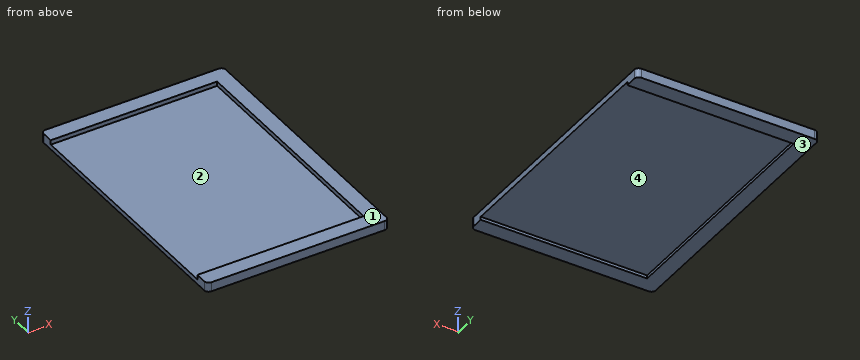
```python
from build123d import *

# Parameters (mm, degrees)
F1_DEPTH = 3.429
F3_DEPTH = 1.651
F5_DEPTH = 1.143


with BuildPart() as f1:
    # F0 (on Top) → F1 (new body)
    with BuildSketch(Plane.XY):
        with BuildLine():
            Line((-31.75, -49.022), (31.75, -49.022))
            ThreePointArc((31.75, -49.022), (32.872532, -48.557032), (33.3375, -47.4345))
            Line((33.3375, -47.4345), (33.3375, 47.4345))
            ThreePointArc((33.3375, 47.4345), (32.872532, 48.557032), (31.75, 49.022))
            Line((31.75, 49.022), (-31.75, 49.022))
            ThreePointArc((-31.75, 49.022), (-32.872532, 48.557032), (-33.3375, 47.4345))
            Line((-33.3375, 47.4345), (-33.3375, -47.4345))
            ThreePointArc((-33.3375, -47.4345), (-32.872532, -48.557032), (-31.75, -49.022))
        make_face()
    extrude(amount=F1_DEPTH)

    # F2 (on face) → F3 (cut)
    with BuildSketch(Plane.XY.offset(3.429)):
        Polygon((-27.6225, -43.307), (27.6225, -43.307), (27.6225, 43.307), (-27.6225, 43.307), (-33.3375, 43.307), (-33.3375, -43.307), align=None)
    extrude(amount=-F3_DEPTH, mode=Mode.SUBTRACT)

    # F4 (on face) → F5 (cut)
    with BuildSketch(Plane(origin=(0, 0, 0), x_dir=(1, 0, 0), z_dir=(0, 0, -1))):
        Polygon((-27.6225, -43.307), (27.6225, -43.307), (33.3375, -43.307), (33.3375, 43.307), (27.6225, 43.307), (-27.6225, 43.307), align=None)
    extrude(amount=-F5_DEPTH, mode=Mode.SUBTRACT)


solid = f1.part
```
Design review of the part built by this model. Coordinates are the model's own, in mm. Face numbers are marked on the shaded views. A direction names the side the tool comes from. Round coordinates to 2 decimals unless told otherwise and drop trailing zeros. Order: outer loops, then holes, each group sorted by start corner. A loop starts at its lowest first (then second) coordinate and runs counter-clockwise, first axis right, second up. Notation, with made-up numbers: (43.25, 3) - (53.25, 3) arc R17 cw to (53.25, 34) - close; hole circle Ø3 at (76.25, 33.5). An arc over 180 degrees is marked (long way). One line per question, with ' | ' between items.
Item 1: Draft analysis for pull direction Y (two halves, no side actions). For the marked faces 3 and 4, state which applies: +Y half, -Y half, draft (parallel to the pull), parting line (faces both ways), or undercut.
Checks:
face 3: draft | face 4: undercut
Item 2: Machinability: for the marked faces 1 and 2, which of the approach directions +Z, -Z, +X, -X, +Y, -Y give a long, thin tool a straight path to every point of the face, cutting with its end or side? Answer none if there is none.
Checks:
face 1: +Z, +X, -X, +Y, -Y | face 2: +Z, -X
Item 3: Take a section at B-B, the plane y = 16. Write out the cut boundary in (x, z), then the cut area to 3 significant figures.
Checks:
outline: (-33.34, 0) - (-27.62, 0) - (-27.62, 1.14) - (33.34, 1.14) - (33.34, 3.43) - (27.62, 3.43) - (27.62, 1.78) - (-33.34, 1.78) - close | area: 58.3 mm²
Item 4: Wall thickness on line 1 (Y direction, x = 27.5, z = 2.45); line 2 (Z direction, x = 7, y = 23); line 3 (X direction, y = 27, z = 2.4): over which ranges is each line inside the solid? List them lowest first. Write a range as [from, to].
Checks:
line 1: [-49.02, -43.31], [43.31, 49.02] | line 2: [1.14, 1.78] | line 3: [27.62, 33.34]
Item 5: For P1, Ø0.5, axis at y = -4, z = 2.5, coming from the -X side; P2, Ø1, axis at x = -10, y = 4.5, coming from the +Z side; P3, Ø0.6, axis at y = 19.5, z = 0.5, coming from the +X side, all flat-tipped, find the tip position at first contact; note any pin that passes through.
Checks:
P1: x = 27.62 | P2: z = 1.78 | P3: x = -27.62
Item 6: Take a section at C-C, the plane x = 19.5. Write out the cut boundary in (y, z), then the cut area to 3 significant figures.
Checks:
outline: (-49.02, 0) - (-43.31, 0) - (-43.31, 1.14) - (43.31, 1.14) - (43.31, 0) - (49.02, 0) - (49.02, 3.43) - (43.31, 3.43) - (43.31, 1.78) - (-43.31, 1.78) - (-43.31, 3.43) - (-49.02, 3.43) - close | area: 94.2 mm²
